Build history of the part. All positions in model axes, mm. A direction names the side the tool comes from. Give positions to 0.01 mm unless a question says otherwise; leave off trailing zeros. Loops run counter-clockwise (first coordinate to the right, second up) from the corner with the lowest first, then second, coordinate; pieces in that order, holes last. Notation, with made-up numbers: M 68,73.5 L 87,73.5 A19 ccw 87,88.5 Z; hole C 79.25,13 d4. An arc over 180 degrees is marked long. Answer in a Markdown table with one row per item. Add a question column.
```python
from build123d import *

# Parameters (mm, degrees)
SKETCH1_R           = 7.875
BOSS_EXTRUDE1_DEPTH = 9.15
BOSS_EXTRUDE4_DEPTH = 11.57
SKETCH12_W          = 8.4
SKETCH12_H          = 5.08
CUT_EXTRUDE36_DEPTH = 3.5
SKETCH13_W          = 8.4
SKETCH13_H          = 5.08
CUT_EXTRUDE37_DEPTH = 3.5
SKETCH14_R          = 6.225
CUT_EXTRUDE38_DEPTH = 4.75
CAVITY1_START       = -7.9
CAVITY1_DEPTH       = 12.3
CAVITY1_START_2     = -8.3
CAVITY1_2_DEPTH     = 0.4
CUT_EXTRUDE40_START = -12.7
CUT_EXTRUDE40_DEPTH = 12.7
CUT_EXTRUDE45_DEPTH = 28.068975322
CUT_EXTRUDE46_DEPTH = 10.5


# Read off the part's stored shape, not the designer's step: Cavity1
with BuildPart() as part:
    # Sketch1 → Boss-Extrude1 (new body)
    with BuildSketch(Plane.XY):
        Circle(SKETCH1_R)
    extrude(amount=BOSS_EXTRUDE1_DEPTH)

    # Sketch2 → Boss-Extrude4 (add)
    with BuildSketch(Plane(origin=(0, 0, 0), x_dir=(-1, 0, 0), z_dir=(0, 0, -1))):
        Polygon((-11.585, 7.874861502), (-11.585, -7.874861502), (0, -7.875), (11.585, -7.874861502), (11.585, 7.874861502), (-9.4146e-05, 7.874999999), align=None)
    extrude(amount=BOSS_EXTRUDE4_DEPTH)

    # Sketch12 → Cut-Extrude36 (cut)
    with BuildSketch(Plane.ZY.offset(11.585)):
        with Locations((-4.2, 0)):
            Rectangle(SKETCH12_W, SKETCH12_H)
    extrude(amount=-CUT_EXTRUDE36_DEPTH, mode=Mode.SUBTRACT)

    # Sketch13 → Cut-Extrude37 (cut)
    with BuildSketch(Plane(origin=(11.585, 0, 0), x_dir=(0, 0, -1), z_dir=(1, 0, 0))):
        with Locations((4.2, 0)):
            Rectangle(SKETCH13_W, SKETCH13_H)
    extrude(amount=-CUT_EXTRUDE37_DEPTH, mode=Mode.SUBTRACT)

    # Sketch14 → Cut-Extrude38 (cut)
    with BuildSketch(Plane.XY.offset(9.15)):
        Circle(SKETCH14_R)
    extrude(amount=-CUT_EXTRUDE38_DEPTH, mode=Mode.SUBTRACT)

    # Cavity1 outline → Cavity1 (cut)
    with BuildSketch(Plane.XY.offset(CAVITY1_START)):
        with BuildLine():
            Line((3.870791195, -2.29498922), (2.460102149, 3.768009742))
            ThreePointArc((2.460102149, 3.768009742), (-1.019783438, 4.382926162), (-3.870791195, 2.29498922))
            Line((-3.870791195, 2.29498922), (-2.460102149, -3.768009742))
            ThreePointArc((-2.460102149, -3.768009742), (1.019783438, -4.382926162), (3.870791195, -2.29498922))
        make_face()
        Polygon((0.567084274, 3.078606085), (1.867874704, -2.51205973), (-0.567084274, -3.078606085), (-1.867874704, 2.51205973), align=None, mode=Mode.SUBTRACT)
    extrude(amount=CAVITY1_DEPTH, mode=Mode.SUBTRACT)

    # Cavity1 2 outline → Cavity1 2 (cut)
    with BuildSketch(Plane.XY.offset(CAVITY1_START_2)):
        with BuildLine():
            ThreePointArc((2.195760692, 3.580312135), (-0.951797876, 4.090731084), (-3.550742498, 2.243262738))
            Line((-3.550742498, 2.243262738), (-2.195760692, -3.580312135))
            ThreePointArc((-2.195760692, -3.580312135), (0.951797876, -4.090731084), (3.550742498, -2.243262738))
            Line((3.550742498, -2.243262738), (2.195760692, 3.580312135))
        make_face()
        Polygon((0.567084274, 3.078606085), (1.867874704, -2.51205973), (-0.567084274, -3.078606085), (-1.867874704, 2.51205973), align=None, mode=Mode.SUBTRACT)
    extrude(amount=CAVITY1_2_DEPTH, mode=Mode.SUBTRACT)

    # Sketch15 → Cut-Extrude40 (cut)
    with BuildSketch(Plane.XY.offset(4.4).offset(CUT_EXTRUDE40_START)):
        Polygon((-1.867874704, 2.51205973), (0.567084274, 3.078606085), (1.867874704, -2.51205973), (-0.567084274, -3.078606085), align=None)
    extrude(amount=CUT_EXTRUDE40_DEPTH, mode=Mode.SUBTRACT)

    # Sketch16 → Cut-Extrude45 (cut, through all)
    with BuildSketch(Plane.ZY.offset(11.585)):
        Polygon((0, 7.874861502), (-11.57, 6.8707), (-11.57, 7.874861502), (-11.57, 8.881300341), (0.174713313, 8.881300341), align=None)
        Polygon((0, -7.874861502), (-11.57, -6.8707), (-11.57, -8.73716659), (0, -8.516935753), align=None)
    extrude(amount=-CUT_EXTRUDE45_DEPTH, mode=Mode.SUBTRACT)

    # Sketch17 → Cut-Extrude46 (cut, symmetric)
    with BuildSketch(Plane(origin=(0, 0, 0), x_dir=(1, 0, 0), z_dir=(0, 1, 0))):
        Polygon((-11.585, 11.57), (11.585, 11.57), (0, 10.22), align=None)
    extrude(amount=CUT_EXTRUDE46_DEPTH, both=True, mode=Mode.SUBTRACT)


solid = part.part
```
(1) Slice it at C-C, the plane y = 0. Give the cut face in (x, z) (3 decimals).
(2) Pin check, flat tips, straight feed: pin 1 (4 mm diameter, centred on y = -0.5, z = -4, fed in from -X) (3 decimals); pin 2 (1 mm diameter, centred on y = 1, z = 0, fed in from +X) (3 decimals); pin 3 (5 mm diameter, centred on y = -3.5, z = 1, fed in from +X) (3 decimals); pin 4 (4 mm diameter, centred on x = -10.5, z = -4, fed in from -Y). Stop position of each tip, or through.
(3) Wall check: line 1 (Y direction, x = 0, z = 5.8) (3 decimals); line 2 (Y direction, x = -10.25, z = -0.5); line 3 (X direction, y = 1, z = 6.75). Give the ranges that are in metal, low to high.
(4) Slice it at D-D, the plane z = -5. Give the cut face in (x, y) (3 decimals).
(5) Slice it at B-B, the plane x = -9. Give the cut face in (y, z).
(6) Pull direction Y, two halves, no side cores. Call faces 1 (the flat face through (-11.585, 3, -6)), 2 (the flat face through (-0.16, -7.38, -5.7)), 3 (the flat face through (-0.16, 7.38, -5.7)), 4 (the flat face through (0, 0, -8.3)): +Y half, -Y half, draft (parallel to the pull), parting line (faces both ways), or undercut.
(7) Slice it at A-A, the plane z = 2. Give the cut face in (x, y) (3 decimals), then the cut area to 3 significant figures.
(8) Tool access for faces 5 (the flat face through (11.585, -3, -6)), 6 (the flat face through (10, 2.54, -4)), 7 (the flat face through (-10, -2.54, -4)), 8 (the cylindrical face through (-4.588, 4.207, 6.808)): list every direction of +Z, -Z, +X, -X, +Y, -Y with a clear straight run to the whole face (end or side of a thin tool).
Solution:
| question | item | result |
|---|---|---|
| 1 | outline | M -11.585,-11.57 L 0,-10.22 L 11.585,-11.57 L 11.585,-8.4 L 8.085,-8.4 L 8.085,0 L 7.875,0 L 7.875,9.15 L 6.225,9.15 L 6.225,4.4 L 3.337,4.4 L 3.337,-7.9 L 3.029,-7.9 L 3.029,-8.3 L -3.029,-8.3 L -3.029,-7.9 L -3.337,-7.9 L -3.337,4.4 L -6.225,4.4 L -6.225,9.15 L -7.875,9.15 L -7.875,0 L -8.085,0 L -8.085,-8.4 L -11.585,-8.4 Z |
| 2 | pin 1 | x = -8.085 |
| 2 | pin 2 | x = 8.085 |
| 2 | pin 3 | x = 11.585 |
| 2 | pin 4 | y = -7.7 |
| 3 | line 1 | -7.875 to -6.225, 6.225 to 7.875 |
| 3 | line 2 | -7.83 to -2.54, 2.54 to 7.83 |
| 3 | line 3 | -7.81 to -6.14, 6.14 to 7.81 |
| 4 | outline | M -11.585,-7.441 L 11.585,-7.441 L 11.585,-2.54 L 8.085,-2.54 L 8.085,2.54 L 11.585,2.54 L 11.585,7.441 L -11.585,7.441 L -11.585,2.54 L -8.085,2.54 L -8.085,-2.54 L -11.585,-2.54 Z; hole M -3.871,2.295 L -2.46,-3.768 A4.5 ccw 3.871,-2.295 L 2.46,3.768 A4.5 ccw Z |
| 5 | outline | M -7.87,0 L -6.9,-11.27 L 6.9,-11.27 L 7.87,0 L 2.54,0 L 2.54,-8.4 L -2.54,-8.4 L -2.54,0 Z |
| 6 | face 1 | draft |
| 6 | face 2 | -Y half |
| 6 | face 3 | +Y half |
| 6 | face 4 | undercut |
| 7 | outline | C 0,0 d15.75; hole M -3.871,2.295 L -2.46,-3.768 A4.5 ccw 3.871,-2.295 L 2.46,3.768 A4.5 ccw Z |
| 7 | area | 142 mm^2 |
| 8 | face 5 | +Z, -Z, +X, +Y, -Y |
| 8 | face 6 | +Z, +X |
| 8 | face 7 | +Z, -X |
| 8 | face 8 | +Z |
